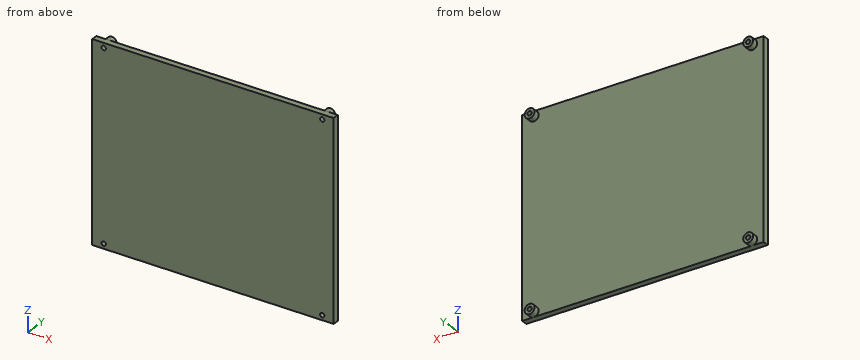
```python
from build123d import *

# Parameters (mm, degrees)
SKETCH1_R           = 1.75
BOSS_EXTRUDE1_DEPTH = 5
SKETCH2_R           = 4
SKETCH2_R_2         = 1.75
BOSS_EXTRUDE2_DEPTH = 5


with BuildPart() as part:
    # Sketch1 → Boss-Extrude1 (new body)
    with BuildSketch(Plane(origin=(0, 0, 0), x_dir=(1, 0, 0), z_dir=(0, 1, 0))):
        Polygon((-92.5, -80), (92.5, -80), (97.5, -80), (97.5, 80), (92.5, 80), (-92.5, 80), (-97.5, 80), (-97.5, -80), align=None)
        with Locations((-88.25, 76)):
            Circle(SKETCH1_R, mode=Mode.SUBTRACT)
        with Locations((88.25, 76)):
            Circle(SKETCH1_R, mode=Mode.SUBTRACT)
        with Locations((88.25, -76)):
            Circle(SKETCH1_R, mode=Mode.SUBTRACT)
        with Locations((-88.25, -76)):
            Circle(SKETCH1_R, mode=Mode.SUBTRACT)
    extrude(amount=BOSS_EXTRUDE1_DEPTH)

    # Sketch2 → Boss-Extrude2 (add)
    with BuildSketch(Plane(origin=(0, 5, 0), x_dir=(1, 0, 0), z_dir=(0, 1, 0))):
        with Locations((-88.25, 76)):
            Circle(SKETCH2_R)
        with Locations((-88.25, 76)):
            Circle(SKETCH2_R_2, mode=Mode.SUBTRACT)
        with Locations((88.25, 76)):
            Circle(SKETCH2_R)
        with Locations((88.25, 76)):
            Circle(SKETCH2_R_2, mode=Mode.SUBTRACT)
        with Locations((88.25, -76)):
            Circle(SKETCH2_R)
        with Locations((88.25, -76)):
            Circle(SKETCH2_R_2, mode=Mode.SUBTRACT)
        with Locations((-88.25, -76)):
            Circle(SKETCH2_R)
        with Locations((-88.25, -76)):
            Circle(SKETCH2_R_2, mode=Mode.SUBTRACT)
    extrude(amount=BOSS_EXTRUDE2_DEPTH)


solid = part.part
```
Source: CAD feature listing. Evaluate the final solid. Frame: model axes, mm. Coordinates: 2 decimals unless noted, no trailing zeros. Write each loop counter-clockwise with the first axis right and the second up, starting at its lowest first coordinate (ties: lowest second). Pieces come first, ordered by that corner, then holes. Notation, with made-up numbers: (73, -30) -> (94, -30) arc R27 ccw to (94, -3) -> close; hole circle Ø11 at (-20, -29.5). An arc over 180 degrees is marked (long way). Return JSON: item names as keys, results as strings. Group by question number.
1) Section query C-C, the plane x = 62. Return loops of the section in (y, z), plus the area to 3 significant figures.
2) Ray query, line 1 along X through (y, z) = (8.25, -76); line 2 along Z through (x, y) = (88.25, 2.5); line 3 along Z through (x, y) = (-88.25, 7.75). Return the intervals inside material, ascending.
3) Section query B-B, the plane z = 14. Return loops of the section in (x, y).
4) Contact query for flat-ended pins moving along their axis: P1, Ø5, axis at x = 34, z = -32.5, coming from the +Y side; P2, Ø2, axis at x = 88.25, z = 76, coming from the +Y side. Output: stop coordinate, or through.
5) Section query A-A, the plane y = 8.25. Return loops of the section in (x, z).
From the geometry:
{
 "1": {"outline": "(0, -80) -> (5, -80) -> (5, 80) -> (0, 80) -> close", "area": "800 mm²"},
 "2": {"line 1": "-92.25 to -90, -86.5 to -84.25, 84.25 to 86.5, 90 to 92.25", "line 2": "-80 to -77.75, -74.25 to 74.25, 77.75 to 80", "line 3": "-80 to -77.75, -74.25 to -72, 72 to 74.25, 77.75 to 80"},
 "3": {"outline": "(-97.5, 0) -> (97.5, 0) -> (97.5, 5) -> (-97.5, 5) -> close"},
 "4": {"P1": "y = 5", "P2": "through"},
 "5": {"outline": "circle Ø8 at (-88.25, -76); circle Ø8 at (-88.25, 76); circle Ø8 at (88.25, -76); circle Ø8 at (88.25, 76); hole circle Ø3.5 at (-88.25, -76); hole circle Ø3.5 at (-88.25, 76); hole circle Ø3.5 at (88.25, -76); hole circle Ø3.5 at (88.25, 76)"}
}
